The listing builds one solid part. Answer for the finished solid, in the listing's coordinates (mm). Coordinates: 2 decimals unless noted, no trailing zeros. Order: outer loops, then holes, each group sorted by start corner. A loop starts at its lowest first (then second) coordinate and runs counter-clockwise, first axis right, second up. Notation, with made-up numbers: M 0.25,82 L 7.25,82 A25 cw 7.25,121 Z; hole C 65.25,-26.75 d11. An arc over 180 degrees is marked long. One line per item, written item: value. Start each with the question number.
Q1. Determine the mould class of faces 1 (the flat face through (37.5, 0, 2)), 2 (the cylindrical face through (21.66, 26.05, 2.47)), 3 (the cylindrical face through (13.497, 0.154, 2.465)), 4 (the cylindrical face through (-34.65, 34.49, 2.54)) for opening direction X: pulls with the +X half, pulls with the -X half, needs draft (parallel to the pull), parting line crosses it, or undercut.
Q2. The part is cut by section A-A on x = 25. Give the vertices of the cut face in (y, z), then the cut area to 3 significant figures.
Q3. Straight lines are drawn through the part: line 1 along Y through (x, z) = (-25, 1.35); line 2 along X through (y, z) = (28, 3.75); line 3 along Y through (x, z) = (24, 2.4). For each, find the intervals that lie inside material, in ascending order. Write a range as [from, to].
Q4. This flat-tipped pin is pushed along its axis until it touches: pin 1 Ø1 at (x, z) = (-29.5, 3.5) entering from +Y. Where does it stop, or does it pass through?
Q5. The part is cut by section C-C on z = 3.3. Give the vertices of the cut face in (x, y), then the cut area to 3 significant figures.
Q6. The part is cut by section B-B on y = 0. Give the vertices of the cut face in (x, z).
```python
from build123d import *

# Parameters (mm, degrees)
SKETCH1_W                = 75
SKETCH1_H                = 75
BOSS_EXTRUDE1_DEPTH      = 5
F_7_0_7_DIAMETER_HOLE2_D = 7
FILLET1_R                = 10
F_7_0_7_DIAMETER_HOLE1_D = 7


with BuildPart() as part:
    # Sketch1 → Boss-Extrude1 (new body)
    with BuildSketch(Plane.XY):
        Rectangle(SKETCH1_W, SKETCH1_H)
    extrude(amount=BOSS_EXTRUDE1_DEPTH)

    # Ø7.0 (7) Diameter Hole2 (through all)
    with Locations(Plane.XY.offset(5)):
        with Locations((-25, 25), (-25, -25), (25, -25), (25, 25)):
            Hole(F_7_0_7_DIAMETER_HOLE2_D / 2)

    # Fillet1
    fillet1_edges = [part.edges().sort_by_distance(p)[0] for p in [
        (-37.5, 37.5, 2.5),
        (37.5, 37.5, 2.5),
        (37.5, -37.5, 2.5),
        (-37.5, -37.5, 2.5),
    ]]
    fillet(fillet1_edges, radius=FILLET1_R)

    # Ø7.0 (7) Diameter Hole1 (through all)
    with Locations(Plane.XY.offset(5)):
        with Locations((10, 0)):
            Hole(F_7_0_7_DIAMETER_HOLE1_D / 2)


solid = part.part
```
Output:
1. face 1: pulls with the +X half
1. face 2: undercut
1. face 3: undercut
1. face 4: pulls with the -X half
2. outline: M -37.5,0 L -28.5,0 L -28.5,5 L -37.5,5 Z; M -21.5,0 L 21.5,0 L 21.5,5 L -21.5,5 Z; M 28.5,0 L 37.5,0 L 37.5,5 L 28.5,5 Z
2. area: 305 mm^2
3. line 1: y = [-37.5, -28.5], [-21.5, 21.5], [28.5, 37.5]
3. line 2: x = [-37.49, -26.8], [-23.2, 23.2], [26.8, 37.49]
3. line 3: y = [-37.5, -28.35], [-21.65, 21.65], [28.35, 37.5]
4. pin 1: stops at y = 37.39
5. outline: M -37.5,-27.5 A10 ccw -27.5,-37.5 L 27.5,-37.5 A10 ccw 37.5,-27.5 L 37.5,27.5 A10 ccw 27.5,37.5 L -27.5,37.5 A10 ccw -37.5,27.5 Z; hole C -25,-25 d7; hole C -25,25 d7; hole C 10,0 d7; hole C 25,-25 d7; hole C 25,25 d7
5. area: 5,350 mm^2
6. outline: M -37.5,0 L 6.5,0 L 6.5,5 L -37.5,5 Z; M 13.5,0 L 37.5,0 L 37.5,5 L 13.5,5 Z
